from build123d import *

# Parameters (mm, degrees)
BOSS_EXTRUDE1_START     = 4
SKETCH3_R               = 60.475
BOSS_EXTRUDE1_DEPTH     = 4
CUT_EXTRUDE1_DEPTH      = 151.434121296
CUT_EXTRUDE1_DEPTH_BACK = 4
SKETCH5_R               = 5.5


with BuildPart() as part:
    # Sketch1 → Revolve1 (revolve)
    with BuildSketch(Plane.XY, mode=Mode.PRIVATE) as revolve1_sk:
        Polygon((53.975, 0), (53.975, 42.5), (57.475, 42.5), (57.475, 82.5), (62.475, 82.5), (62.475, 118.56), (65.475, 118.56), (65.475, 79.5), (60.475, 79.5), (60.475, 0), align=None)
    revolve(revolve1_sk.sketch.rotate(Axis((0, 0, 0), (0, 1, 0)), 90), axis=Axis((0, 0, 0), (0, 1, 0)))

    # Sketch3 → Boss-Extrude1 (add)
    with BuildSketch(Plane.XZ.offset(BOSS_EXTRUDE1_START)):
        with Locations(Location((0, 0, 0), (0, 0, 270))):
            Circle(SKETCH3_R)
    extrude(amount=-BOSS_EXTRUDE1_DEPTH)

    # Sketch5 → Cut-Extrude1 (cut, two sides: drawn at the far end of the back side and taken through both)
    with BuildSketch(Plane.XY.offset(-CUT_EXTRUDE1_DEPTH_BACK)):
        with Locations(Location((0, 15.5, 0), (0, 0, 180))):
            Circle(SKETCH5_R)
    extrude(amount=CUT_EXTRUDE1_DEPTH + CUT_EXTRUDE1_DEPTH_BACK, mode=Mode.SUBTRACT)


solid = part.part
Geometry check sheet. Reference: the model listing, model coordinates, mm. A direction names the side the tool comes from. Round coordinates to 2 decimals unless told otherwise and drop trailing zeros. Write each loop counter-clockwise with the first axis right and the second up, starting at its lowest first coordinate (ties: lowest second). Pieces come first, ordered by that corner, then holes.
Item 1: Section check D-D (y = 5.5). Record the boundary of the cut face in (x, z) (3 decimals).
Determined:
outline: circle Ø120.95 at (0, 0); hole circle Ø107.95 at (0, 0)
Item 2: Section check C-C (x = 14). Record the boundary of the cut face in (y, z), plus the area to 3 significant figures.
Determined:
outline: (-4, -58.83) - (79.5, -58.83) - (79.5, -63.96) - (118.56, -63.96) - (118.56, -60.89) - (82.5, -60.89) - (82.5, -55.74) - (42.5, -55.74) - (42.5, -52.13) - (0, -52.13) - (0, 52.13) - (42.5, 52.13) - (42.5, 55.74) - (82.5, 55.74) - (82.5, 60.89) - (118.56, 60.89) - (118.56, 63.96) - (79.5, 63.96) - (79.5, 58.83) - (-4, 58.83) - close
area: 1,540 mm2
Item 3: Section check A-A (x = 0). Record the boundary of the cut face in (y, z) (3 decimals).
Determined:
outline: (-4, -60.475) - (79.5, -60.475) - (79.5, -65.475) - (118.56, -65.475) - (118.56, -62.475) - (82.5, -62.475) - (82.5, -57.475) - (42.5, -57.475) - (42.5, -53.975) - (0, -53.975) - (0, 53.975) - (10, 53.975) - (10, 60.475) - (-4, 60.475) - close; (21, 53.975) - (42.5, 53.975) - (42.5, 57.475) - (82.5, 57.475) - (82.5, 62.475) - (118.56, 62.475) - (118.56, 65.475) - (79.5, 65.475) - (79.5, 60.475) - (21, 60.475) - close
Item 4: Section check B-B (z = 0). Record the boundary of the cut face in (x, y) (3 decimals), plus the area to 3 significant figures.
Determined:
outline: (-65.475, 79.5) - (-60.475, 79.5) - (-60.475, -4) - (60.475, -4) - (60.475, 79.5) - (65.475, 79.5) - (65.475, 118.56) - (62.475, 118.56) - (62.475, 82.5) - (57.475, 82.5) - (57.475, 42.5) - (53.975, 42.5) - (53.975, 0) - (-53.975, 0) - (-53.975, 42.5) - (-57.475, 42.5) - (-57.475, 82.5) - (-62.475, 82.5) - (-62.475, 118.56) - (-65.475, 118.56) - close
area: 1,520 mm2
Item 5: Go/stop test with flat-tipped pins: pin 1 Ø2 at (y, z) = (81.5, -12) entering from -X; pin 2 Ø5 at (x, y) = (8, 19) entering from -Z; pin 3 Ø4 at (x, z) = (-38, -38.5) entering from +Y. Record where each tip stops, or that it passes through.
Determined:
pin 1: stops at x = -64.54
pin 2: stops at z = -60.22
pin 3: stops at y = 42.5
Item 6: Access from +Z, -Z, +X, -X, +Y, -Y to the whole of each face (thin tool, end or side, straight path). Record for faces 4 (the face through (-19.67, 98.76, -62.45)), 5 (the face through (58, 79.5, -19)), 6 (the face through (-51.4, 42.5, -17.3)).
Determined:
face 4: +Y, -Y
face 5: -Y
face 6: +Y
Item 7: Mould release check, pull along Z, two halves, no side actions. Record for faces 1 (the face through (-23.162, 37.166, -55.864)), 2 (the face through (-61.943, 100.782, 8.133)), 3 (the face through (1.19, 20.87, 57.04)): +Z half, -Z half, draft (parallel to the pull), parting line (faces both ways), or undercut.
Determined:
face 1: parting line
face 2: undercut
face 3: draft
Item 8: Material ranges on line 1 along X through (y, z) = (22, 0) (3 decimals); line 2 along Y through (x, z) = (0, 55.5); line 3 along X through (y, z) = (97.5, 0) (3 decimals), recorded low to high.
Determined:
line 1: x = -60.475 to -53.975, 53.975 to 60.475
line 2: y = -4 to 10, 21 to 42.5
line 3: x = -65.475 to -62.475, 62.475 to 65.475
